Here's how the part is built. I have some questions about the finished solid (model axes, mm). Round coordinates to 2 decimals unless told otherwise and drop trailing zeros. Order: outer loops, then holes, each group sorted by start corner. A loop starts at its lowest first (then second) coordinate and runs counter-clockwise, first axis right, second up.
```python
from build123d import *

# Parameters (mm, degrees)
ESBO_O1_W                = 195
ESBO_O1_H                = 120
RESSALTO_EXTRUS_O1_DEPTH = 3
FILETE1_R                = 20
FILETE2_R                = 20
FILETE3_R                = 20
FILETE4_R                = 20
ESBO_O2_W                = 10
ESBO_O2_H                = 3.5
CORTE_EXTRUS_O1_DEPTH    = 229.984715647
CORTE_EXTRUS_O2_DEPTH    = 229.984715647
ESBO_O4_R                = 4.75
ESBO_O4_W                = 8.5
ESBO_O4_H                = 13.5
CORTE_EXTRUS_O3_DEPTH    = 229.984715647
ESBO_O5_R                = 5
ESBO_O5_R_2              = 2
ESBO_O5_W                = 10
ESBO_O5_H                = 40
CORTE_EXTRUS_O4_DEPTH    = 229.984715647


with BuildPart() as part:
    # Esboço1 → Ressalto-extrusão1 (new body)
    with BuildSketch(Plane(origin=(0, 0, 0), x_dir=(1, 0, 0), z_dir=(0, 1, 0))):
        with Locations((97.5, 60)):
            Rectangle(ESBO_O1_W, ESBO_O1_H)
    extrude(amount=RESSALTO_EXTRUS_O1_DEPTH)

    # Filete1
    filete1_edges = [part.edges().sort_by_distance(p)[0] for p in [
        (0, 1.5, 0),
    ]]
    fillet(filete1_edges, radius=FILETE1_R)

    # Filete2
    filete2_edges = [part.edges().sort_by_distance(p)[0] for p in [
        (195, 1.5, 0),
    ]]
    fillet(filete2_edges, radius=FILETE2_R)

    # Filete3
    filete3_edges = [part.edges().sort_by_distance(p)[0] for p in [
        (195, 1.5, -120),
    ]]
    fillet(filete3_edges, radius=FILETE3_R)

    # Filete4
    filete4_edges = [part.edges().sort_by_distance(p)[0] for p in [
        (0, 1.5, -120),
    ]]
    fillet(filete4_edges, radius=FILETE4_R)

    # Esboço2 → Corte-extrusão1 (cut, through all)
    with BuildSketch(Plane(origin=(0, 3, 0), x_dir=(1, 0, 0), z_dir=(0, 1, 0))):
        with Locations((110, 1.75)):
            Rectangle(ESBO_O2_W, ESBO_O2_H)
        with Locations((110, 118.25)):
            Rectangle(ESBO_O2_W, ESBO_O2_H)
        with Locations((110, 23.25)):
            Rectangle(ESBO_O2_W, ESBO_O2_H)
        with Locations((110, 96.75)):
            Rectangle(ESBO_O2_W, ESBO_O2_H)
        with Locations((155.5, 23.25)):
            Rectangle(ESBO_O2_W, ESBO_O2_H)
        with Locations((185, 23.25)):
            Rectangle(ESBO_O2_W, ESBO_O2_H)
        with Locations((155.5, 96.75)):
            Rectangle(ESBO_O2_W, ESBO_O2_H)
        with Locations((185, 96.75)):
            Rectangle(ESBO_O2_W, ESBO_O2_H)
    extrude(amount=-CORTE_EXTRUS_O1_DEPTH, mode=Mode.SUBTRACT)

    # Esboço3 → Corte-extrusão2 (cut, through all)
    with BuildSketch(Plane(origin=(0, 3, 0), x_dir=(1, 0, 0), z_dir=(0, 1, 0))):
        with BuildLine():
            Line((164, 87), (164, 77))
            ThreePointArc((164, 77), (162.25, 75.25), (160.5, 77))
            Line((160.5, 77), (160.5, 87))
            ThreePointArc((160.5, 87), (162.25, 88.75), (164, 87))
        make_face()
        with BuildLine():
            Line((164, 43), (164, 33))
            ThreePointArc((164, 33), (162.25, 31.25), (160.5, 33))
            Line((160.5, 33), (160.5, 43))
            ThreePointArc((160.5, 43), (162.25, 44.75), (164, 43))
        make_face()
        with BuildLine():
            Line((90, 43), (90, 33))
            ThreePointArc((90, 33), (88.25, 31.25), (86.5, 33))
            Line((86.5, 33), (86.5, 43))
            ThreePointArc((86.5, 43), (88.25, 44.75), (90, 43))
        make_face()
        with BuildLine():
            Line((90, 88.75), (90, 78.75))
            ThreePointArc((90, 78.75), (88.25, 77), (86.5, 78.75))
            Line((86.5, 78.75), (86.5, 88.75))
            ThreePointArc((86.5, 88.75), (88.25, 90.5), (90, 88.75))
        make_face()
    extrude(amount=-CORTE_EXTRUS_O2_DEPTH, mode=Mode.SUBTRACT)

    # Esboço4 → Corte-extrusão3 (cut, through all)
    with BuildSketch(Plane(origin=(0, 3, 0), x_dir=(1, 0, 0), z_dir=(0, 1, 0))):
        with Locations(Location((110, 77, 0), (0, 0, 270))):
            Circle(ESBO_O4_R)
        with Locations((110.75, 54.25)):
            Rectangle(ESBO_O4_W, ESBO_O4_H)
    extrude(amount=-CORTE_EXTRUS_O3_DEPTH, mode=Mode.SUBTRACT)

    # Esboço5 → Corte-extrusão4 (cut, through all)
    with BuildSketch(Plane(origin=(0, 3, 0), x_dir=(1, 0, 0), z_dir=(0, 1, 0))):
        with Locations(Location((40, 95, 0), (0, 0, 270))):
            Circle(ESBO_O5_R)
        with Locations(Location((20, 77, 0), (0, 0, 270))):
            Circle(ESBO_O5_R_2)
        with Locations(Location((20, 43, 0), (0, 0, 270))):
            Circle(ESBO_O5_R_2)
        with Locations((43, 60)):
            Rectangle(ESBO_O5_W, ESBO_O5_H)
    extrude(amount=-CORTE_EXTRUS_O4_DEPTH, mode=Mode.SUBTRACT)


solid = part.part
```
1. I'm going to push flat-ended pins straight in: P1, Ø0.9, axis at x = 112, y = 1.5, coming from the -Z side; P2, Ø10, axis at x = 92.5, z = -21, coming from the -Y side; P3, Ø1.5, axis at x = 185.5, y = 1, coming from the -Z side; P4, Ø1.5, axis at x = 183.5, y = 1.5, coming from the -Z side. Where does each tip first touch, or does it pass through?
Evaluation:
P1: stops at z = -116.5
P2: stops at y = 0
P3: stops at z = -117.46
P4: stops at z = -118.44
2. If we mould it in two halves opening along X, with no side actions, what happens to faces 1 (the cylindrical face through (188.986, 1.521, -5.703)), 2 (the cylindrical face through (6.014, 1.521, -114.297)), 3 (the cylindrical face through (105.363, 1.521, -78.03))? For each: released by +X, released by -X, zero draft, split by the parting line, or undercut.
Evaluation:
face 1: released by +X
face 2: released by -X
face 3: undercut
3. If we section it at A-A, the plane x = 40: Write out the boundary of the cut face in (y, z).
Evaluation:
outline: (0, -120) - (3, -120) - (3, -100) - (0, -100) - close; (0, -90) - (3, -90) - (3, -80) - (0, -80) - close; (0, -40) - (3, -40) - (3, 0) - (0, 0) - close
4. If we section it at B-B, the plane y = 1.45: State how many separate pieces and enclosed holes the cut face has, and give its area (3 significant figures).
Evaluation:
separate pieces: 1
enclosed holes: 16
area: 21,900 mm2
5. If we section it at C-C, the plane z = -111: Write out the boundary of the cut face in (x, y).
Evaluation:
outline: (3.3, 0) - (191.7, 0) - (191.7, 3) - (3.3, 3) - close
6. I need wall thicknesses on probe 1 along X at (y, z) = (1.25, -82); probe 2 along X at (y, z) = (1.7, -43); probe 3 along Z at (x, y) = (108.5, 1.55). Which ranges of each line are inside material? Lowest first, please.
Evaluation:
probe 1: x = 0 to 86.5, 90 to 160.5, 164 to 195
probe 2: x = 0 to 18, 22 to 38, 48 to 86.5, 90 to 160.5, 164 to 195
probe 3: z = -116.5 to -98.5, -95 to -81.51, -72.49 to -61, -47.5 to -25, -21.5 to -3.5
